from build123d import *

# Parameters (mm, degrees)
F0_W      = 38.1
F0_H      = 38.1
F1_DEPTH  = 38.1
F6_DEPTH  = 38.1
F8_DEPTH  = 38.1
F9_W      = 25.4
F9_H      = 7.617908
F9_H_2    = 7.62
F10_DEPTH = 38.1


with BuildPart() as f1:
    # F0 (on Front) → F1 (new body)
    with BuildSketch(Plane.XZ):
        with Locations((19.05, 19.05)):
            Rectangle(F0_W, F0_H)
    extrude(amount=F1_DEPTH)

    # F5 (on offset) → F6 (cut)
    with BuildSketch(Plane.YZ.offset(38.1)):
        Polygon((-11.43, 14.589625), (-6.35, 38.1), (-31.75, 38.1), (-26.67, 15.875), (-21.59, 28.575), (-16.51, 28.575), align=None)
        Polygon((-31.75, 0), (-38.1, 38.1), (-38.1, 0), align=None)
        Polygon((-25.4, 0), (-12.7, 0), (-19.05, 15.875), align=None)
        Polygon((-6.35, 0), (0, 0), (0, 38.1), align=None)
    extrude(amount=-F6_DEPTH, mode=Mode.SUBTRACT)

    # F7 (on offset) → F8 (cut)
    with BuildSketch(Plane.XZ.offset(38.1)):
        Polygon((0, 38.1), (0, 0), (6.35, 38.1), align=None)
        Polygon((25.4, 38.1), (12.7, 38.1), (19.05, 22.225), align=None)
        Polygon((11.43, 16.466031), (6.35, 0), (31.75, 0), (26.67, 16.466031), (21.59, 9.525), (16.51, 9.525), align=None)
        Polygon((31.75, 38.1), (38.1, 0), (38.1, 38.1), align=None)
    extrude(amount=-F8_DEPTH, mode=Mode.SUBTRACT)

    # F9 (on offset) → F10 (cut)
    with BuildSketch(Plane.XY.offset(38.1)):
        with Locations((25.4, -11.428954)):
            Rectangle(F9_W, F9_H)
        with Locations((12.7, -26.667908)):
            Rectangle(F9_W, F9_H_2)
    extrude(amount=-F10_DEPTH, mode=Mode.SUBTRACT)


solid = f1.part
Model file for the job. Use its own axes, mm. A direction names the side the tool comes from. Round coordinates to 2 decimals unless told otherwise and drop trailing zeros. Order: outer loops, then holes, each group sorted by start corner. A loop starts at its lowest first (then second) coordinate and runs counter-clockwise, first axis right, second up. Notation, with made-up numbers: M 77.5,70 L 98.5,70 A15 cw 98.5,74 Z; hole C 81,-19.75 d3. An arc over 180 degrees is marked long. Write each question's results on one line, items separated by ' | '. Start each with the question number.
(1) Drop flat-ended pins along their axis: pin 1 (0.9 mm diameter, centred on x = 20.5, y = -5.5, fed in from -Z) (3 decimals); pin 2 (10 mm diameter, centred on y = -14.5, z = 31.5, fed in from -X); pin 3 (20.5 mm diameter, centred on x = 23.5, z = 14.5, fed in from +Y) (3 decimals). Give the stop position or say it passes through.
(2) Which spindle directions (+Z, -Z, +X, -X, +Y, -Y) get a long thin tool onto all of the face, cutting with end or side? Do faces 5 (the face through (3, -9, 0)), 6 (the face through (28, -19, 28.575)), 7 (the face through (13, -30.478, 20)), 8 (the face through (32, -17.1, 11)). Say none if no direction does.
(3) Saw through at D-D, the plane y = -10. Give the cut face in (x, z).
(4) Probe probe 1 along Y at (x, z) = (5.5, 8); probe 2 along Y at (x, z) = (15, 15); probe 3 along Y at (x, z) = (16, 25). List the from-to ranges inside material, lowest first. Write a range as from..to.
(5) Saw through at B-B, the plane z = 21.5. Give the cut face in (x, y).
(6) Two-plate mould, pull along X, no slides. Class faces 1 (the face through (32.6, -22.2, 8)), 2 (the face through (12.7, -14, 18)), 3 (the face through (25.4, -28, 20)), 4 (the face through (14.006, -32.068, 12.947)): pulls with the +X half, pulls with the -X half, needs draft (parallel to the pull), parting line crosses it, or undercut.
(7) Saw through at C-C, the plane z = 8. Give the cut face in (x, y).
(8) Saw through at A-A, the plane z = 29.5. Give the cut face in (x, y), then the cut area to 3 significant figures.
Established:
1) pin 1: stops at z = 9.525 | pin 2: stops at x = 4.45 | pin 3: stops at y = -2.225
2) face 5: -Z, +X, -X, +Y, -Y | face 6: +Z, +X, -X | face 7: +Z, -Z, -X | face 8: -Z, +X, -X
3) outline: M 0,0 L 6.35,0 L 11.43,16.47 L 12.7,14.73 L 12.7,21.21 L 3.53,21.21 Z
4) probe 1: y = -33.08..-30.48, -22.86..-22.2, -15.9..-5.02 | probe 2: y = -34.25..-30.48, -22.86..-19.4, -18.7..-15.24, -7.62..-3.85 | probe 3: y = -35.92..-30.48, -22.86..-15.24, -7.62..-2.18
5) outline: M 3.58,-35.33 L 34.52,-35.33 L 34.52,-27.96 L 25.4,-27.96 L 25.4,-30.48 L 3.58,-30.48 Z; M 3.58,-22.86 L 25.4,-22.86 L 25.4,-24.42 L 34.52,-24.42 L 34.52,-15.24 L 12.7,-15.24 L 12.7,-13.94 L 3.58,-13.94 Z; M 3.58,-9.94 L 12.7,-9.94 L 12.7,-7.62 L 34.52,-7.62 L 34.52,-2.77 L 3.58,-2.77 Z
6) face 1: needs draft | face 2: pulls with the +X half | face 3: pulls with the -X half | face 4: undercut
7) outline: M 1.33,-33.08 L 8.82,-33.08 L 8.82,-30.48 L 1.33,-30.48 Z; M 1.33,-22.86 L 8.82,-22.86 L 8.82,-22.2 L 1.33,-22.2 Z; M 1.33,-15.9 L 8.82,-15.9 L 8.82,-5.02 L 1.33,-5.02 Z; M 29.28,-33.08 L 36.77,-33.08 L 36.77,-22.2 L 29.28,-22.2 Z; M 29.28,-15.9 L 36.77,-15.9 L 36.77,-15.24 L 29.28,-15.24 Z; M 29.28,-7.62 L 36.77,-7.62 L 36.77,-5.02 L 29.28,-5.02 Z
8) outline: M 4.92,-36.67 L 16.14,-36.67 L 16.14,-30.48 L 4.92,-30.48 Z; M 4.92,-8.21 L 12.7,-8.21 L 12.7,-7.62 L 16.14,-7.62 L 16.14,-1.43 L 4.92,-1.43 Z; M 21.96,-36.67 L 33.18,-36.67 L 33.18,-29.78 L 25.4,-29.78 L 25.4,-30.48 L 21.96,-30.48 Z; M 21.96,-7.62 L 33.18,-7.62 L 33.18,-1.43 L 21.96,-1.43 Z | area: 288 mm^2
